from build123d import *

# Parameters (mm, degrees)
CUT_EXTRUDE2_DEPTH      = 19.920887928
CUT_EXTRUDE2_DEPTH_BACK = 19.920887928
SKETCH3_R               = 3
SKETCH2_R               = 4
CUT_EXTRUDE1_DEPTH      = 2.5
CUT_EXTRUDE4_START      = 2.5
SKETCH4_R               = 4
CUT_EXTRUDE4_DEPTH      = 2.5


with BuildPart() as part:
    # Sketch1 → Revolve1 (revolve)
    with BuildSketch(Plane.XY):
        Polygon((-7, 0), (-7, 9), (-5.5, 9), (-5.5, 6.07), (5.5, 6.07), (5.5, 9), (7, 9), (7, 0), align=None)
    revolve(axis=Axis((7, 0, 0), (-1, 0, 0)))

    # Sketch3 → Cut-Extrude2 (cut, two sides: drawn at the far end of the back side and taken through both)
    with BuildSketch(Plane(origin=(7, 0, 0), x_dir=(0, 0, -1), z_dir=(1, 0, 0)).offset(-CUT_EXTRUDE2_DEPTH_BACK)):
        with Locations(Location((0, 0, 0), (0, 0, 90))):
            Circle(SKETCH3_R)
    extrude(amount=CUT_EXTRUDE2_DEPTH + CUT_EXTRUDE2_DEPTH_BACK, mode=Mode.SUBTRACT)

    # Sketch2 → Cut-Extrude1 (cut)
    with BuildSketch(Plane(origin=(-7, 0, 18.209055513), x_dir=(0, 0, 1), z_dir=(-1, 0, 0))):
        with Locations(Location((-18.209055513, 0, 0), (0, 0, 270))):
            Circle(SKETCH2_R)
    extrude(amount=-CUT_EXTRUDE1_DEPTH, mode=Mode.SUBTRACT)

    # Sketch4 → Cut-Extrude4 (cut)
    with BuildSketch(Plane(origin=(7, 0, 11.209055513), x_dir=(0, 0, 1), z_dir=(-1, 0, 0)).offset(CUT_EXTRUDE4_START)):
        with Locations(Location((-11.209055513, 0, 0), (0, 0, 270))):
            Circle(SKETCH4_R)
    extrude(amount=-CUT_EXTRUDE4_DEPTH, mode=Mode.SUBTRACT)


solid = part.part
CAD build for the part. Positions are in the model's coordinates, mm. A direction names the side the tool comes from. Round coordinates to 2 decimals unless told otherwise and drop trailing zeros. Order: outer loops, then holes, each group sorted by start corner. A loop starts at its lowest first (then second) coordinate and runs counter-clockwise, first axis right, second up. Notation, with made-up numbers: M 40.25,41.25 L 59.25,41.25 A15 cw 59.25,66.25 Z; hole C -28.5,27 d3. An arc over 180 degrees is marked long. Use one line per item in the form item = value.
Q1. Which spindle directions (+Z, -Z, +X, -X, +Y, -Y) get a long thin tool onto all of the face, cutting with end or side? Do faces 1 (the cylindrical face through (6.26, -1.172, -8.923)), 2 (the cylindrical face through (-5.768, 0.867, -3.905)), 3 (the flat face through (-5.5, 2, 6)), 4 (the flat face through (-7, -2, 4)), 5 (the cylindrical face through (5.732, 0.867, -3.905)). Say none if no direction does.
Recorded:
face_1 = +X, -X
face_2 = -X
face_3 = none
face_4 = +Z, -Z, -X, +Y, -Y
face_5 = +X
Q2. Flat gauge pins, fed straight in: P1, Ø2.5, axis at y = 1, z = 1.5, coming from the +X side; P2, Ø9, axis at y = 1, z = -2, coming from the -X side; P3, Ø1.5, axis at x = 4, y = 5, coming from the +Z side; P4, Ø1.5, axis at x = 3.5, z = -5, coming from the -Y side. Where does each tip first touch, or does it go through?
Recorded:
P1 = 4.5
P2 = -7
P3 = 4.33
P4 = -4.33
Q3. Two-plate mould, pull along Z, no slides. Class faces 6 (the flat face through (4.5, -1, 3)), 7 (the cylindrical face through (-6.24, -1.172, -8.923)), 8 (the flat face through (7, 2, 4)): +Z half, -Z half, draft (parallel to the pull), parting line (faces both ways), or undercut.
Recorded:
face_6 = undercut
face_7 = parting line
face_8 = draft
Q4. Probe L1, parallel to Z at x = 6.25, y = 0; L2, parallel to Y at x = 0.5, z = 0; L3, parallel to X at y = 2, z = -6.25. List the from-to ranges inside material, lowest first.
Recorded:
L1 = -9 to -4, 4 to 9
L2 = -6.07 to -3, 3 to 6.07
L3 = -7 to -5.5, 5.5 to 7
Q5. Saw through at C-C on x = 2. Give the cut face in (y, z), then the cut area to 3 significant figures.
Recorded:
outline = C 0,0 d12.14; hole C 0,0 d6
area = 87.5 mm^2
Q6. Saw through at A-A on y = 0. Give the cut face in (x, z), then the cut area to 3 significant figures.
Recorded:
outline = M -7,-9 L -5.5,-9 L -5.5,-6.07 L 5.5,-6.07 L 5.5,-9 L 7,-9 L 7,-4 L 4.5,-4 L 4.5,-3 L -4.5,-3 L -4.5,-4 L -7,-4 Z; M -7,4 L -4.5,4 L -4.5,3 L 4.5,3 L 4.5,4 L 7,4 L 7,9 L 5.5,9 L 5.5,6.07 L -5.5,6.07 L -5.5,9 L -7,9 Z
area = 93.5 mm^2
Q7. Saw through at D-D on z = -3.5. Give the cut face in (x, y), then the cut area to 3 significant figures.
Recorded:
outline = M -7,-8.29 L -5.5,-8.29 L -5.5,-4.96 L 5.5,-4.96 L 5.5,-8.29 L 7,-8.29 L 7,-1.94 L 4.5,-1.94 L 4.5,1.94 L 7,1.94 L 7,8.29 L 5.5,8.29 L 5.5,4.96 L -5.5,4.96 L -5.5,8.29 L -7,8.29 L -7,1.94 L -4.5,1.94 L -4.5,-1.94 L -7,-1.94 Z
area = 139 mm^2
